Job drawing, mm, ordinate dimensions from the low corner. One solid piece. A direction names the side the tool comes from. Give positions to 0.01 mm unless a question says otherwise; leave off trailing zeros. Order: outer loops, then holes, each group sorted by start corner. A loop starts at its lowest first (then second) coordinate and runs counter-clockwise, first axis right, second up.
Item 1: Two-plate mould, pull along X, no slides. Class the marked faces 1, 2, 3 and 4: released by +X, released by -X, zero draft, split by the parting line, or undercut.
Item 2: Wall check: L1, parallel to X at y = 934, z = 588; L2, parallel to X at y = 326.5, z = 102; L3, parallel to Z at x = 1280, y = 145.5. Give the ranges that are in metal, low to high.
Item 3: Band-saw the part on D-D on y = 1038. Give the cut face in (x, z), plus the area to 3 significant figures.
Item 4: Band-saw the part on C-C on y = 237. Give the cut face in (x, z).
Item 5: Band-saw the part on A-A on z = 445. Give the cut face in (x, y).
Item 6: Flat gauge pins, fed straight in: P1, Ø6, axis at x = 1455.5, z = 564.5, coming from the -Y side; P2, Ø1, axis at y = 342.5, z = 389, coming from the -X side. Where does each tip first touch, or does it go through?
Item 7: Band-saw the part on B-B on y = 716. Give the cut face in (x, z).
Item 8: Which spindle directions (+Z, -Z, +X, -X, +Y, -Y) get a long thin tool onto all of the face, cutting with end or side? Do the marked faces 5 and 6. Say none if no direction does.
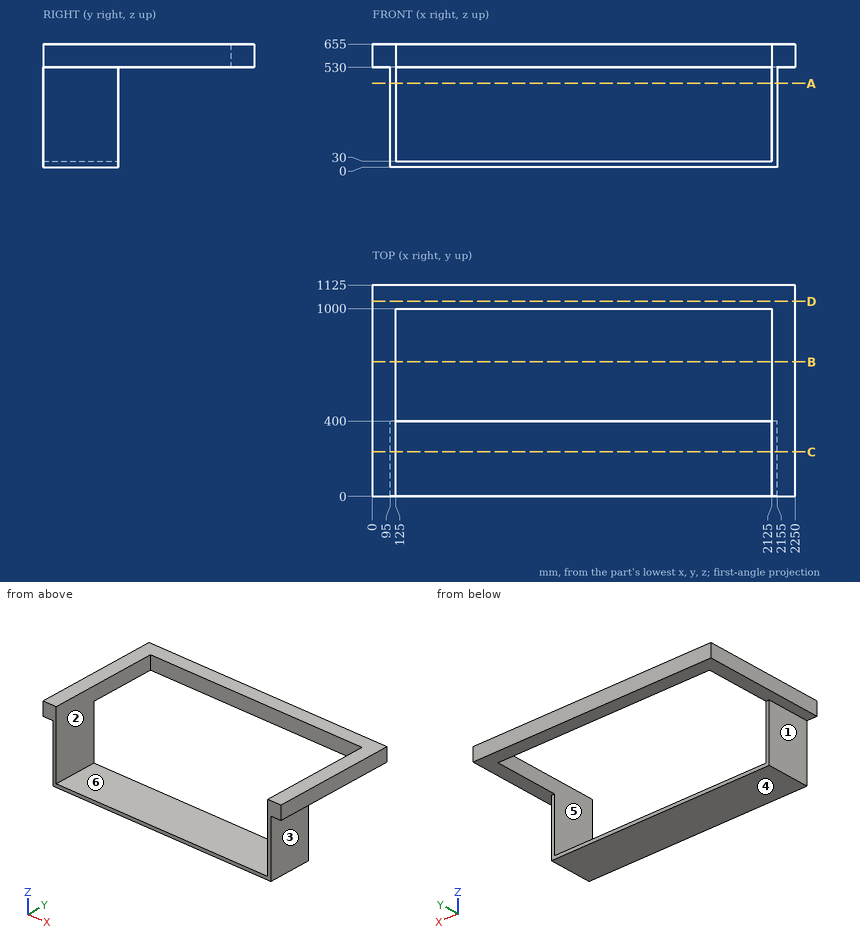
The answers:
1. face 1: released by -X
1. face 2: undercut
1. face 3: released by +X
1. face 4: zero draft
2. L1: x = 0 to 125, 2125 to 2250
2. L2: x = 95 to 125, 2125 to 2155
2. L3: z = 0 to 30
3. outline: (0, 530) - (2250, 530) - (2250, 655) - (0, 655) - close
3. area: 281,000 mm2
4. outline: (0, 530) - (95, 530) - (95, 0) - (2155, 0) - (2155, 530) - (2250, 530) - (2250, 655) - (2125, 655) - (2125, 30) - (125, 30) - (125, 655) - (0, 655) - close
5. outline: (95, 0) - (125, 0) - (125, 400) - (95, 400) - close; (2125, 0) - (2155, 0) - (2155, 400) - (2125, 400) - close
6. P1: stops at y = 1000
6. P2: stops at x = 95
7. outline: (0, 530) - (125, 530) - (125, 655) - (0, 655) - close; (2125, 530) - (2250, 530) - (2250, 655) - (2125, 655) - close
8. face 5: +Z, -Y
8. face 6: +Z, +Y, -Y
